from build123d import *

# Parameters (mm, degrees)
SKETCH1_W           = 140
SKETCH1_H           = 70
BOSS_EXTRUDE1_DEPTH = 10
FILLET1_R           = 10
SKETCH2_R           = 2.75
CUT_EXTRUDE1_DEPTH  = 79.89866919
SKETCH3_R           = 4
CUT_EXTRUDE2_DEPTH  = 79.89866919
SKETCH4_R           = 2.625
SKETCH4_R_2         = 1.5
CUT_EXTRUDE3_DEPTH  = 79.89866919
SKETCH5_W           = 60
SKETCH5_H           = 46
CUT_EXTRUDE4_DEPTH  = 79.89866919
FILLET3_R           = 10


with BuildPart() as part:
    # Sketch1 → Boss-Extrude1 (new body)
    with BuildSketch(Plane(origin=(0, 0, 0), x_dir=(1, 0, 0), z_dir=(0, 1, 0))):
        Rectangle(SKETCH1_W, SKETCH1_H)
    extrude(amount=BOSS_EXTRUDE1_DEPTH)

    # Fillet1
    fillet1_edges = [part.edges().sort_by_distance(p)[0] for p in [
        (70, 5, 35),
        (-70, 5, 35),
        (-70, 5, -35),
        (70, 5, -35),
    ]]
    fillet(fillet1_edges, radius=FILLET1_R)

    # Sketch2 → Cut-Extrude1 (cut, through all)
    with BuildSketch(Plane(origin=(0, 10, 0), x_dir=(1, 0, 0), z_dir=(0, 1, 0))):
        with Locations(Location((-60, -25, 0), (0, 0, 270))):
            Circle(SKETCH2_R)
        with Locations(Location((-60, 25, 0), (0, 0, 90))):
            Circle(SKETCH2_R)
        with Locations(Location((60, -25, 0), (0, 0, 90))):
            Circle(SKETCH2_R)
        with Locations(Location((60, 25, 0), (0, 0, 270))):
            Circle(SKETCH2_R)
    extrude(amount=-CUT_EXTRUDE1_DEPTH, mode=Mode.SUBTRACT)

    # Sketch3 → Cut-Extrude2 (cut, through all)
    with BuildSketch(Plane(origin=(0, 10, 0), x_dir=(1, 0, 0), z_dir=(0, 1, 0))):
        with Locations(Location((-50, 4, 0), (0, 0, 270))):
            Circle(SKETCH3_R)
        with Locations(Location((50, 4, 0), (0, 0, 90))):
            Circle(SKETCH3_R)
    extrude(amount=-CUT_EXTRUDE2_DEPTH, mode=Mode.SUBTRACT)

    # Sketch4 → Cut-Extrude3 (cut, through all)
    with BuildSketch(Plane(origin=(0, 10, 0), x_dir=(1, 0, 0), z_dir=(0, 1, 0))):
        with Locations(Location((-63, -7, 0), (0, 0, 270))):
            Circle(SKETCH4_R)
        with Locations(Location((-37, -7, 0), (0, 0, 270))):
            Circle(SKETCH4_R)
        with Locations(Location((37, -7, 0), (0, 0, 270))):
            Circle(SKETCH4_R)
        with Locations(Location((63, -7, 0), (0, 0, 270))):
            Circle(SKETCH4_R)
        with Locations(Location((-63, 0.25, 0), (0, 0, 270))):
            Circle(SKETCH4_R_2)
        with Locations(Location((-37, 0.25, 0), (0, 0, 270))):
            Circle(SKETCH4_R_2)
        with Locations(Location((37, 0.25, 0), (0, 0, 270))):
            Circle(SKETCH4_R_2)
        with Locations(Location((63, 0.25, 0), (0, 0, 270))):
            Circle(SKETCH4_R_2)
    extrude(amount=-CUT_EXTRUDE3_DEPTH, mode=Mode.SUBTRACT)

    # Sketch5 → Cut-Extrude4 (cut, through all)
    with BuildSketch(Plane(origin=(0, 10, 0), x_dir=(1, 0, 0), z_dir=(0, 1, 0))):
        Rectangle(SKETCH5_W, SKETCH5_H)
    extrude(amount=-CUT_EXTRUDE4_DEPTH, mode=Mode.SUBTRACT)

    # Fillet3
    fillet3_edges = [part.edges().sort_by_distance(p)[0] for p in [
        (-30, 5, 23),
        (-30, 5, -23),
        (30, 5, -23),
        (30, 5, 23),
    ]]
    fillet(fillet3_edges, radius=FILLET3_R)


solid = part.part
The model under review builds one solid part; all positions refer to its coordinate system, in mm. A direction names the side the tool comes from. Coordinates: 2 decimals unless noted, no trailing zeros. Write each loop counter-clockwise with the first axis right and the second up, starting at its lowest first coordinate (ties: lowest second). Pieces come first, ordered by that corner, then holes. Notation, with made-up numbers: (6, -23.5) -> (49, -23.5) arc R21 ccw to (49, -17.5) -> close; hole circle Ø7 at (7, -39.5). An arc over 180 degrees is marked (long way). Answer in a Markdown table with one row per item.
1. Draft analysis for pull direction X (two halves, no side actions). For faces 1 (the cylindrical face through (-62.727, 5.07, -24.642)), 2 (the cylindrical face through (-61.226, 5.07, 5.065)), 3 (the flat face through (70, 5, 0)), 4 (the flat face through (-1, 5, -35)), state which applies: +X half, -X half, draft (parallel to the pull), parting line (faces both ways), or undercut.
Answers below:
| item | result |
|---|---|
| face 1 | undercut |
| face 2 | undercut |
| face 3 | +X half |
| face 4 | draft |
2. We need section C-C, the plane z = 7. State the section outline as (x, y) points (3 decimals), and give its area (3 significant figures).
Answers below:
| item | result |
|---|---|
| outline | (-70, 0) -> (-65.625, 0) -> (-65.625, 10) -> (-70, 10) -> close; (-60.375, 0) -> (-39.625, 0) -> (-39.625, 10) -> (-60.375, 10) -> close; (-34.375, 0) -> (-30, 0) -> (-30, 10) -> (-34.375, 10) -> close; (30, 0) -> (34.375, 0) -> (34.375, 10) -> (30, 10) -> close; (39.625, 0) -> (60.375, 0) -> (60.375, 10) -> (39.625, 10) -> close; (65.625, 0) -> (70, 0) -> (70, 10) -> (65.625, 10) -> close |
| area | 590 mm^2 |
3. We need section A-A, the plane z = -4. State the section outline as (x, y) points.
Answers below:
| item | result |
|---|---|
| outline | (-70, 0) -> (-54, 0) -> (-54, 10) -> (-70, 10) -> close; (-46, 0) -> (-30, 0) -> (-30, 10) -> (-46, 10) -> close; (30, 0) -> (46, 0) -> (46, 10) -> (30, 10) -> close; (54, 0) -> (70, 0) -> (70, 10) -> (54, 10) -> close |
4. We need section B-B, the plane x = 50. State the section outline as (y, z) points, and give its area (3 significant figures).
Answers below:
| item | result |
|---|---|
| outline | (0, -35) -> (10, -35) -> (10, -8) -> (0, -8) -> close; (0, 0) -> (10, 0) -> (10, 35) -> (0, 35) -> close |
| area | 620 mm^2 |
5. We need section D-D, the plane y = 8.5. Give the number of separate pieces and of enclosed holes in the cut face, and give its area (3 significant figures).
Answers below:
| item | result |
|---|---|
| separate pieces | 1 |
| enclosed holes | 15 |
| area | 6,730 mm^2 |
6. Wall thickness on probe 1 along X at (y, z) = (4, -25); probe 2 along X at (y, z) = (4.5, 7) (3 decimals); probe 3 along X at (y, z) = (4.5, -10.5): over which ranges is each line inside the solid? List them lowest first. Write a range as [from, to].
Answers below:
| item | result |
|---|---|
| probe 1 | x = [-70, -62.75], [-57.25, 57.25], [62.75, 70] |
| probe 2 | x = [-70, -65.625], [-60.375, -39.625], [-34.375, -30], [30, 34.375], [39.625, 60.375], [65.625, 70] |
| probe 3 | x = [-70, -30], [30, 70] |
7. For faces 5 (the flat face through (-30, 5, 0)), 6 (the cylindrical face through (-67.15, 5.07, -31.99)), list the 3-axis set-ups (+Z, -Z, +X, -X, +Y, -Y) from which the entire face can be reached by the end or side of a thin tool; tool diameter is ignored.
Answers below:
| item | result |
|---|---|
| face 5 | +Y, -Y |
| face 6 | -Z, -X, +Y, -Y |
